Verification items for the finished model (mm, model axes). A direction names the side the tool comes from. Give positions to 0.01 mm unless a question says otherwise; leave off trailing zeros. Order: outer loops, then holes, each group sorted by start corner. A loop starts at its lowest first (then second) coordinate and runs counter-clockwise, first axis right, second up. Notation, with made-up numbers: (76.5, -18) -> (134.5, -18) arc R22 cw to (134.5, 6) -> close; hole circle Ø2 at (20.25, 36.25). An arc over 180 degrees is marked (long way). Write each question's results on one line, items separated by ' | '. Start each with the question number.
1. Material ranges on L1, parallel to Y at x = 1.9, z = -10; L2, parallel to X at y = 1, z = -15; L3, parallel to Z at x = 16.5, y = 5.25, recorded low to high. Write a range as from..to.
2. Mould release check, pull along Y, two halves, no side actions. Record for faces 3 (the face through (4, 9, -3)), 4 (the face through (0, 2.1, -12.1)), 5 (the face through (7.43, -1.06, -1.52)): +Y half, -Y half, draft (parallel to the pull), parting line (faces both ways), or undercut.
3. Depth check by flat-ended pin: pin 1 Ø9 at (y, z) = (3, -9.5) entering from +X; pin 2 Ø4 at (x, y) = (17, 5) entering from -Z. Enter the tip coordinate at first touch or a pass-through.
4. Cross-section at A-A, the plane z = -10. Enter the section's corners in (x, y), then the cut area to 3 significant figures.
5. Cross-section at B-B, the plane y = 0. Enter the section's corners in (x, z).
6. Cross-section at C-C, the plane x = 10.75. Enter the section's corners in (y, z), then the cut area to 3 significant figures.
7. Set-up check for faces 1 (the face through (12.4, 2.1, -3)), 2 (the face through (12.4, -1.9, 0)): record each of +Z, -Z, +X, -X, +Y, -Y from which the full face is reachable in a straight line by a thin tool's end or side.
8. Cross-section at D-D, the plane y = 7.75. Enter the section's corners in (x, z).
from build123d import *

# Parameters (mm, degrees)
BOSS_EXTRUDE1_DEPTH = 9
SKETCH2_R           = 2.78
CUT_EXTRUDE1_DEPTH  = 28.748873851
SKETCH3_R           = 2.78
CUT_EXTRUDE2_DEPTH  = 28.748873851


with BuildPart() as part:
    # Sketch1 → Boss-Extrude1 (new, symmetric)
    with BuildSketch(Plane(origin=(0, 0, 0), x_dir=(1, 0, 0), z_dir=(0, 1, 0))):
        with BuildLine():
            Line((0, 0), (0, 20))
            ThreePointArc((0, 20), (2.121320344, 19.121320344), (3, 17))
            Line((3, 17), (3, 5.5))
            ThreePointArc((3, 5.5), (3.732233047, 3.732233047), (5.5, 3))
            Line((5.5, 3), (17, 3))
            ThreePointArc((17, 3), (19.121320344, 2.121320344), (20, 0))
            Line((20, 0), (0, 0))
        make_face()
    extrude(amount=BOSS_EXTRUDE1_DEPTH, both=True)

    # Sketch2 → Cut-Extrude1 (cut, through all)
    with BuildSketch(Plane(origin=(0, 0, -3), x_dir=(-1, 0, 0), z_dir=(0, 0, -1))):
        with Locations((-10, 0)):
            Circle(SKETCH2_R)
    extrude(amount=-CUT_EXTRUDE1_DEPTH, mode=Mode.SUBTRACT)

    # Sketch3 → Cut-Extrude2 (cut, through all)
    with BuildSketch(Plane(origin=(3, 0, 0), x_dir=(0, 0, -1), z_dir=(1, 0, 0))):
        with Locations((10, 0)):
            Circle(SKETCH3_R)
    extrude(amount=-CUT_EXTRUDE2_DEPTH, mode=Mode.SUBTRACT)


solid = part.part
Results below:
1) L1: y = -9..-2.78, 2.78..9 | L2: x = 0..3 | L3: z = -3..0
2) face 3: +Y half | face 4: draft | face 5: undercut
3) pin 1: stops at x = 3.05 | pin 2: stops at z = -3
4) outline: (0, -9) -> (3, -9) -> (3, -2.78) -> (0, -2.78) -> close; (0, 2.78) -> (3, 2.78) -> (3, 9) -> (0, 9) -> close | area: 37.3 mm²
5) outline: (0, -20) arc R3 ccw to (3, -17) -> (3, -12.78) -> (0, -12.78) -> close; (0, -7.22) -> (3, -7.22) -> (3, -5.5) arc R2.5 cw to (5.5, -3) -> (7.22, -3) -> (7.22, 0) -> (0, 0) -> close; (12.78, -3) -> (17, -3) arc R3 ccw to (20, 0) -> (12.78, 0) -> close
6) outline: (-9, -3) -> (-2.68, -3) -> (-2.68, 0) -> (-9, 0) -> close; (2.68, -3) -> (9, -3) -> (9, 0) -> (2.68, 0) -> close | area: 37.9 mm²
7) face 1: -Z, +X, +Y, -Y | face 2: +Z, +X, -X, +Y, -Y
8) outline: (0, -20) arc R3 ccw to (3, -17) -> (3, -5.5) arc R2.5 cw to (5.5, -3) -> (17, -3) arc R3 ccw to (20, 0) -> (0, 0) -> close
